Here's how the part is built. I have some questions about the finished solid (model axes, mm). A direction names the side the tool comes from. Round coordinates to 2 decimals unless told otherwise and drop trailing zeros. Loops run counter-clockwise (first coordinate to the right, second up) from the corner with the lowest first, then second, coordinate; pieces in that order, holes last. Notation, with made-up numbers: (19, 55) -> (60, 55) arc R13 ccw to (60, 75) -> close; hole circle Ø2 at (-27, 17). An arc over 180 degrees is marked (long way). Use one line per item in the form item = value. Start each with the question number.
Item 1: If we section it at B-B (y = 52): Write out the boundary of the cut face in (x, z) (1 decimal).
Item 2: If we section it at C-C (x = 14): Write out the boundary of the cut face in (y, z) (1 decimal).
Item 3: If I drill on L1, parallel to Y at x = -2, z = 37 (3 decimals); L2, parallel to Y at x = 2, z = 14.5, over which ranges is the centre line in solid material (lowest first)? Write a range as [from, to].
Item 4: I'm going to push flat-ended pins straight in: pin 1 Ø3 at (y, z) = (-9.5, 50) entering from -X (3 decimals); pin 2 Ø4.5 at (x, z) = (-58.5, 9) entering from -Y; pin 3 Ø1.5 at (x, z) = (23.5, 36) entering from +Y (3 decimals). Where does each tip first touch, or does it pass through?
Item 5: If we section it at A-A (z = 54.5): Write out the boundary of the cut face in (x, y) (3 decimals), then the cut area to 3 significant figures.
Item 6: Thinking about a two-plate mould opening in X: for faces 1 (the face through (-1, -50.125, 40)), 2 (the face through (-50.125, -1, 40)), 3 (the face through (-63, 0, 12)), 4 (the face through (-60, -20, 8)), which applies, released by +X, released by -X, zero draft, split by the parting line, or undercut?
Item 7: If we section it at D-D (y = -32): Write out the boundary of the cut face in (x, z) (3 decimals).
Item 8: For faces 5 (the face through (46.07, 46.18, 24.65)), 6 (the face through (52, 1, 8)), 7 (the face through (50.125, -46, 75)), 8 (the face through (52, 1, 50)), 9 (the face through (20, 60, 8)), which set-ups out of +Z, -Z, +X, -X, +Y, -Y let a thin tool reach every point of the face, with its end or its side?
```python
from build123d import *

# Parameters (mm, degrees)
SKETCH1_W                                    = 108.25
SKETCH1_H                                    = 108.25
SKETCH1_W_2                                  = 100.25
SKETCH1_H_2                                  = 100.25
BASE_DEPTH                                   = 50
CHAMFER_2_SIZE                               = 8
WALL_BRACE_DEPTH                             = 20
WALL_BRACE_PATTERN_COUNT                     = 4
LATTICE_SUPPORT_ARM_DEPTH                    = 50
LATTICE_SUPPORT_ARM_MIRROR_AT_THE_SE_3_DEPTH = 50
ARCHES_1_REACH                               = 168.395
ARCHES_2_REACH                               = 168.395


with BuildPart() as part:
    # Sketch1 → Base (new body)
    with BuildSketch(Plane.XY):
        Rectangle(SKETCH1_W, SKETCH1_H)
        Rectangle(SKETCH1_W_2, SKETCH1_H_2, mode=Mode.SUBTRACT)
    extrude(amount=BASE_DEPTH)

    # Chamfer 2
    chamfer_2_edges = [part.edges().sort_by_distance(p)[0] for p in [
        (50.125, -50.125, 25),
        (50.125, 50.125, 25),
        (-50.125, 50.125, 25),
        (-50.125, -50.125, 25),
    ]]
    chamfer(chamfer_2_edges, length=CHAMFER_2_SIZE)

    # Sketch3 → Wall-Brace (add, symmetric)
    with BuildSketch(Plane(origin=(0, 0, 0), x_dir=(1, 0, 0), z_dir=(0, 1, 0))):
        Polygon((54.125, 0), (63, -6.65625), (63, -16.65625), (59, -16.65625), (59, -8.65625), (54.125, -5), align=None)
    wall_brace = extrude(amount=WALL_BRACE_DEPTH, both=True)

    # Wall-Brace-Pattern: Wall-Brace ×4 about axis
    wall_brace_pattern_axis = Axis((0, 0, 0), (0, 0, 1))
    for i in range(1, WALL_BRACE_PATTERN_COUNT):
        add(wall_brace.rotate(wall_brace_pattern_axis, i * 360 / WALL_BRACE_PATTERN_COUNT))

    # Sketch4 → Lattice-Support-Arm (add)
    with BuildSketch(Plane.XY.offset(50)):
        Polygon((-50.125, 42.125), (-54.125, 42.125), (-54.125, 54.125), (-42.125, 54.125), (-42.125, 50.125), (-50.125, 50.125), align=None)
    lattice_support_arm = extrude(amount=LATTICE_SUPPORT_ARM_DEPTH)

    # Lattice-Support-Arm-Mirror: Lattice-Support-Arm across plane
    add(lattice_support_arm.mirror(Plane(origin=(0, 0, 0), x_dir=(0, 0, 1), z_dir=(1, 0, 0))))

    # Lattice-Support-Arm-Mirror at the second: Lattice-Support-Arm across plane
    add(lattice_support_arm.mirror(Plane.ZX))

    # Lattice-Support-Arm-Mirror at the se 2 → Lattice-Support-Arm-Mirror at the se 3 (add)
    with BuildSketch(Plane(origin=(0, 0, 50), x_dir=(-1, 0, 0), z_dir=(0, 0, 1))):
        Polygon((-50.125, 42.125), (-54.125, 42.125), (-54.125, 54.125), (-42.125, 54.125), (-42.125, 50.125), (-50.125, 50.125), align=None)
    extrude(amount=LATTICE_SUPPORT_ARM_MIRROR_AT_THE_SE_3_DEPTH)

    # Arches-1: up to this face of the body (flat: up to its plane)
    arches_1_end = Plane(part.part.faces().sort_by_distance((-54.125, 0, 35.058479532))[0])
    # Sketch5 → Arches-1 (cut, up to the picked face)
    with BuildSketch(Plane.ZY.offset(-54.125), mode=Mode.PRIVATE) as arches_1_sk1:
        with BuildLine():
            Line((8, 45), (8, -45))
            ThreePointArc((8, -45), (36.205505282, 0), (8, 45))
        make_face()
    arches_1_tool1 = split(extrude(arches_1_sk1.sketch, amount=ARCHES_1_REACH, mode=Mode.PRIVATE), bisect_by=arches_1_end, keep=Keep.BOTH, mode=Mode.PRIVATE)
    add(arches_1_tool1.solids().sort_by(Axis((54.125, 0, 19.609008), (-1, 0, 0)))[0], mode=Mode.SUBTRACT)

    # Arches-2: up to this face of the body (flat: up to its plane)
    arches_2_end = Plane(part.part.faces().sort_by_distance((0, -54.125, 35.058479532))[0])
    # Sketch6 → Arches-2 (cut, up to the picked face)
    with BuildSketch(Plane(origin=(0, 54.125, 0), x_dir=(1, 0, 0), z_dir=(0, 1, 0)), mode=Mode.PRIVATE) as arches_2_sk1:
        with BuildLine():
            Line((-45, -8), (45, -8))
            ThreePointArc((45, -8), (0, -36.205505282), (-45, -8))
        make_face()
    arches_2_tool1 = split(extrude(arches_2_sk1.sketch, amount=-ARCHES_2_REACH, mode=Mode.PRIVATE), bisect_by=arches_2_end, keep=Keep.BOTH, mode=Mode.PRIVATE)
    add(arches_2_tool1.solids().sort_by(Axis((0, 54.125, 19.609008), (0, -1, 0)))[0], mode=Mode.SUBTRACT)


solid = part.part
```
Values found:
q1.outline = (-54.1, 0) -> (54.1, 0) -> (54.1, 100) -> (42.1, 100) -> (42.1, 50) -> (-42.1, 50) -> (-42.1, 100) -> (-54.1, 100) -> close; hole (-45, 8) -> (45, 8) arc R50 ccw to start
q2.outline = (-63, 6.7) -> (-54.1, 0) -> (-50.1, 0) -> (-50.1, 8) -> (-54.1, 8) -> (-54.1, 5) -> (-59, 8.7) -> (-59, 16.7) -> (-63, 16.7) -> close; (-54.1, 34.2) -> (-50.1, 34.2) -> (-50.1, 50) -> (-54.1, 50) -> close; (50.1, 0) -> (54.1, 0) -> (63, 6.7) -> (63, 16.7) -> (59, 16.7) -> (59, 8.7) -> (54.1, 5) -> (54.1, 8) -> (50.1, 8) -> close; (50.1, 34.2) -> (54.1, 34.2) -> (54.1, 50) -> (50.1, 50) -> close
q3.L1 = [-54.125, -50.125], [50.125, 54.125]
q3.L2 = [-63, -59], [59, 63]
q4.pin_1 = -54.125
q4.pin_2 = -20
q4.pin_3 = 54.125
q5.outline = (-54.125, -54.125) -> (-42.125, -54.125) -> (-42.125, -50.125) -> (-50.125, -50.125) -> (-50.125, -42.125) -> (-54.125, -42.125) -> close; (-54.125, 42.125) -> (-50.125, 42.125) -> (-50.125, 50.125) -> (-42.125, 50.125) -> (-42.125, 54.125) -> (-54.125, 54.125) -> close; (42.125, -54.125) -> (54.125, -54.125) -> (54.125, -42.125) -> (50.125, -42.125) -> (50.125, -50.125) -> (42.125, -50.125) -> close; (42.125, 50.125) -> (50.125, 50.125) -> (50.125, 42.125) -> (54.125, 42.125) -> (54.125, 54.125) -> (42.125, 54.125) -> close
q5.area = 320 mm2
q6.face_1 = undercut
q6.face_2 = undercut
q6.face_3 = released by -X
q6.face_4 = zero draft
q7.outline = (-54.125, 0) -> (-50.125, 0) -> (-50.125, 8) -> (-54.125, 8) -> close; (-54.125, 24.624) -> (-50.125, 24.624) -> (-50.125, 50) -> (-54.125, 50) -> close; (50.125, 0) -> (54.125, 0) -> (54.125, 8) -> (50.125, 8) -> close; (50.125, 24.624) -> (54.125, 24.624) -> (54.125, 50) -> (50.125, 50) -> close
q8.face_5 = +Z, -Z
q8.face_6 = none
q8.face_7 = +Z
q8.face_8 = +Z, +X, -X
q8.face_9 = +Z, -Z, +X, +Y
